Verification items for the finished model (mm, model axes). Face numbers are marked on the shaded views. A direction names the side the tool comes from. Coordinates: 2 decimals unless noted, no trailing zeros. Order: outer loops, then holes, each group sorted by start corner. A loop starts at its lowest first (then second) coordinate and runs counter-clockwise, first axis right, second up. Notation, with made-up numbers: M 7,-11 L 48,-11 A19 cw 48,5 Z; hole C -28,2 d4. An arc over 180 degrees is marked long. Use one line per item in the form item = value. Start each with the question number.
```python
from build123d import *

# Parameters (mm, degrees)
F1_DEPTH = 12
F0_W     = 22.75
F0_H     = 12
F2_DEPTH = 29
F3_DEPTH = 8
F4_W     = 10
F4_H     = 4.5
F5_DEPTH = 5.5


with BuildPart() as f1:
    # F0 (on Top) → F1 (new body)
    with BuildSketch(Plane.XY):
        with BuildLine():
            Line((37.5, -50), (34.2948445635, -50))
            ThreePointArc((34.2948445635, -50), (37.0207144417, -53.2303243355), (39.4433779545, -56.6938577061))
            ThreePointArc((39.4433779545, -56.6938577061), (37.9956721228, -53.4851272883), (37.5, -50))
        make_face()
        with BuildLine():
            Line((-34.2948445635, -50), (-37.5, -50))
            ThreePointArc((-37.5, -50), (-37.9956721876, -53.4851275115), (-39.4433782034, -56.6938580986))
            ThreePointArc((-39.4433782034, -56.6938580986), (-37.0207145834, -53.2303245197), (-34.2948445635, -50))
        make_face()
        with BuildLine():
            ThreePointArc((-39.443378119, 56.6938579655), (-37.9956721656, 53.4851274358), (-37.5, 50))
            Line((-37.5, 50), (-34.2948445635, 50))
            ThreePointArc((-34.2948445635, 50), (-37.0207145354, 53.2303244572), (-39.443378119, 56.6938579655))
        make_face()
        with BuildLine():
            Line((50, -34.2948445635), (50, -37.5))
            ThreePointArc((50, -37.5), (53.4851274351, -37.9956721654), (56.6938579643, -39.4433781183))
            ThreePointArc((56.6938579643, -39.4433781183), (53.2303244566, -37.020714535), (50, -34.2948445635))
        make_face()
        with BuildLine():
            Line((50, 37.5), (50, 34.2948445635))
            ThreePointArc((50, 34.2948445635), (53.2303242081, 37.0207143438), (56.6938574347, 39.4433777825))
            ThreePointArc((56.6938574347, 39.4433777825), (53.485127134, 37.995672078), (50, 37.5))
        make_face()
        with BuildLine():
            ThreePointArc((-56.6938576889, -39.4433779436), (-53.4851272786, -37.9956721199), (-50, -37.5))
            Line((-50, -37.5), (-50, -34.2948445635))
            ThreePointArc((-50, -34.2948445635), (-53.2303243274, -37.0207144356), (-56.6938576889, -39.4433779436))
        make_face()
        with BuildLine():
            ThreePointArc((-56.6938579169, 39.4433780882), (-53.2303244344, 37.0207145179), (-50, 34.2948445635))
            Line((-50, 34.2948445635), (-50, 37.5))
            ThreePointArc((-50, 37.5), (-53.4851274082, 37.9956721576), (-56.6938579169, 39.4433780882))
        make_face()
        with BuildLine():
            ThreePointArc((37.5, 50), (41.1611652352, 41.1611652352), (50, 37.5))
            Line((50, 37.5), (50, 44))
            ThreePointArc((50, 44), (45.7573593129, 45.7573593129), (44, 50))
            Line((44, 50), (37.5, 50))
        make_face()
        with BuildLine():
            Line((50, 44), (50, 37.5))
            ThreePointArc((50, 37.5), (53.485127134, 37.995672078), (56.6938574347, 39.4433777825))
            ThreePointArc((56.6938574347, 39.4433777825), (60.952698707, 43.9760153525), (62.5, 50))
            ThreePointArc((62.5, 50), (53.4152371074, 62.0243983426), (39.3662151199, 56.5705874261))
            ThreePointArc((39.3662151199, 56.5705874261), (37.9756016574, 53.4152371074), (37.5, 50))
            Line((37.5, 50), (44, 50))
            ThreePointArc((44, 50), (50, 56), (56, 50))
            ThreePointArc((56, 50), (54.2426406871, 45.7573593129), (50, 44))
        make_face()
        with BuildLine():
            Line((44, -50), (37.5, -50))
            ThreePointArc((37.5, -50), (37.9956721228, -53.4851272883), (39.4433779545, -56.6938577061))
            ThreePointArc((39.4433779545, -56.6938577061), (53.4851272883, -62.0043278772), (62.5, -50))
            ThreePointArc((62.5, -50), (60.9526988581, -43.9760156272), (56.6938579643, -39.4433781183))
            ThreePointArc((56.6938579643, -39.4433781183), (53.4851274351, -37.9956721654), (50, -37.5))
            Line((50, -37.5), (50, -44))
            ThreePointArc((50, -44), (54.2426406871, -45.7573593129), (56, -50))
            ThreePointArc((56, -50), (50, -56), (44, -50))
        make_face()
        with BuildLine():
            ThreePointArc((-39.4433782034, -56.6938580986), (-37.9956721876, -53.4851275115), (-37.5, -50))
            Line((-37.5, -50), (-44, -50))
            ThreePointArc((-44, -50), (-54.2426406871, -54.2426406871), (-50, -44))
            Line((-50, -44), (-50, -37.5))
            ThreePointArc((-50, -37.5), (-53.4851272786, -37.9956721199), (-56.6938576889, -39.4433779436))
            ThreePointArc((-56.6938576889, -39.4433779436), (-58.8388349363, -58.8388345933), (-39.4433782034, -56.6938580986))
        make_face()
        with BuildLine():
            ThreePointArc((-56.6938579169, 39.4433780882), (-53.4851274082, 37.9956721576), (-50, 37.5))
            Line((-50, 37.5), (-50, 44))
            ThreePointArc((-50, 44), (-54.2426406871, 54.2426406871), (-44, 50))
            Line((-44, 50), (-37.5, 50))
            ThreePointArc((-37.5, 50), (-37.9956721656, 53.4851274358), (-39.443378119, 56.6938579655))
            ThreePointArc((-39.443378119, 56.6938579655), (-58.8388347851, 58.8388347445), (-56.6938579169, 39.4433780882))
        make_face()
        with BuildLine():
            Line((22.75, 12), (22.75, 0))
            Line((22.75, 0), (35, 0))
            ThreePointArc((35, 0), (38.9140035649, 18.7158780427), (50, 34.2948445635))
            Line((50, 34.2948445635), (50, 37.5))
            ThreePointArc((50, 37.5), (41.1611652352, 41.1611652352), (37.5, 50))
            Line((37.5, 50), (34.2948445635, 50))
            ThreePointArc((34.2948445635, 50), (18.7158780427, 38.9140035649), (0, 35))
            Line((0, 35), (0, 12))
            Line((0, 12), (22.75, 12))
        make_face()
        with BuildLine():
            ThreePointArc((0, -35), (18.7158780427, -38.9140035649), (34.2948445635, -50))
            Line((34.2948445635, -50), (37.5, -50))
            ThreePointArc((37.5, -50), (41.1611652352, -41.1611652352), (50, -37.5))
            Line((50, -37.5), (50, -34.2948445635))
            ThreePointArc((50, -34.2948445635), (38.9140035649, -18.7158780427), (35, 0))
            Line((35, 0), (22.75, 0))
            Line((22.75, 0), (22.75, -12))
            Line((22.75, -12), (0, -12))
            Line((0, -12), (0, -35))
        make_face()
        with BuildLine():
            ThreePointArc((-50, -37.5), (-41.1611652352, -41.1611652352), (-37.5, -50))
            Line((-37.5, -50), (-34.2948445635, -50))
            ThreePointArc((-34.2948445635, -50), (-18.7158780427, -38.9140035649), (0, -35))
            Line((0, -35), (0, -12))
            Line((0, -12), (-22.75, -12))
            Line((-22.75, -12), (-22.75, 0))
            Line((-22.75, 0), (-35, 0))
            ThreePointArc((-35, 0), (-38.9140035649, -18.7158780427), (-50, -34.2948445635))
            Line((-50, -34.2948445635), (-50, -37.5))
        make_face()
        with BuildLine():
            Line((-50, 37.5), (-50, 34.2948445635))
            ThreePointArc((-50, 34.2948445635), (-38.9140035649, 18.7158780427), (-35, 0))
            Line((-35, 0), (-22.75, 0))
            Line((-22.75, 0), (-22.75, 12))
            Line((-22.75, 12), (0, 12))
            Line((0, 12), (0, 35))
            ThreePointArc((0, 35), (-18.7158780427, 38.9140035649), (-34.2948445635, 50))
            Line((-34.2948445635, 50), (-37.5, 50))
            ThreePointArc((-37.5, 50), (-41.1611652352, 41.1611652352), (-50, 37.5))
        make_face()
        with BuildLine():
            Line((-44, -50), (-37.5, -50))
            ThreePointArc((-37.5, -50), (-41.1611652352, -41.1611652352), (-50, -37.5))
            Line((-50, -37.5), (-50, -44))
            ThreePointArc((-50, -44), (-45.7573593129, -45.7573593129), (-44, -50))
        make_face()
        with BuildLine():
            Line((-50, 44), (-50, 37.5))
            ThreePointArc((-50, 37.5), (-41.1611652352, 41.1611652352), (-37.5, 50))
            Line((-37.5, 50), (-44, 50))
            ThreePointArc((-44, 50), (-45.7573593129, 45.7573593129), (-50, 44))
        make_face()
        with BuildLine():
            ThreePointArc((50, -37.5), (41.1611652352, -41.1611652352), (37.5, -50))
            Line((37.5, -50), (44, -50))
            ThreePointArc((44, -50), (45.7573593129, -45.7573593129), (50, -44))
            Line((50, -44), (50, -37.5))
        make_face()
        with BuildLine():
            ThreePointArc((39.2932775844, 56.4586962355), (36.935506218, 53.1198826695), (34.2948445635, 50))
            Line((34.2948445635, 50), (37.5, 50))
            ThreePointArc((37.5, 50), (37.9756016574, 53.4152371074), (39.3662151199, 56.5705874261))
            Line((39.3662151199, 56.5705874261), (39.2932775844, 56.4586962355))
        make_face()
    extrude(amount=F1_DEPTH)

    # F0 (on Top) → F2 (join)
    with BuildSketch(Plane.XY):
        with Locations((-11.375, 6)):
            Rectangle(F0_W, F0_H)
        with Locations((11.375, 6)):
            Rectangle(F0_W, F0_H)
        with Locations((11.375, -6)):
            Rectangle(F0_W, F0_H)
        with Locations((-11.375, -6)):
            Rectangle(F0_W, F0_H)
    extrude(amount=F2_DEPTH)

    # F0 (on Top) → F3 (join)
    with BuildSketch(Plane.XY):
        with BuildLine():
            ThreePointArc((-44, 50), (-54.2426406871, 54.2426406871), (-50, 44))
            Line((-50, 44), (-50, 47.5))
            ThreePointArc((-50, 47.5), (-51.767766953, 51.767766953), (-47.5, 50))
            Line((-47.5, 50), (-44, 50))
        make_face()
        with BuildLine():
            Line((-50, 47.5), (-50, 44))
            ThreePointArc((-50, 44), (-45.7573593129, 45.7573593129), (-44, 50))
            Line((-44, 50), (-47.5, 50))
            ThreePointArc((-47.5, 50), (-48.232233047, 48.232233047), (-50, 47.5))
        make_face()
        with BuildLine():
            Line((50, 47.5), (50, 44))
            ThreePointArc((50, 44), (54.2426406871, 45.7573593129), (56, 50))
            ThreePointArc((56, 50), (50, 56), (44, 50))
            Line((44, 50), (47.5, 50))
            ThreePointArc((47.5, 50), (50, 52.5), (52.5, 50))
            ThreePointArc((52.5, 50), (51.767766953, 48.232233047), (50, 47.5))
        make_face()
        with BuildLine():
            ThreePointArc((44, 50), (45.7573593129, 45.7573593129), (50, 44))
            Line((50, 44), (50, 47.5))
            ThreePointArc((50, 47.5), (48.232233047, 48.232233047), (47.5, 50))
            Line((47.5, 50), (44, 50))
        make_face()
        with BuildLine():
            ThreePointArc((50, -44), (45.7573593129, -45.7573593129), (44, -50))
            Line((44, -50), (47.5, -50))
            ThreePointArc((47.5, -50), (48.232233047, -48.232233047), (50, -47.5))
            Line((50, -47.5), (50, -44))
        make_face()
        with BuildLine():
            Line((47.5, -50), (44, -50))
            ThreePointArc((44, -50), (50, -56), (56, -50))
            ThreePointArc((56, -50), (54.2426406871, -45.7573593129), (50, -44))
            Line((50, -44), (50, -47.5))
            ThreePointArc((50, -47.5), (51.767766953, -48.232233047), (52.5, -50))
            ThreePointArc((52.5, -50), (50, -52.5), (47.5, -50))
        make_face()
        with BuildLine():
            Line((-47.5, -50), (-44, -50))
            ThreePointArc((-44, -50), (-45.7573593129, -45.7573593129), (-50, -44))
            Line((-50, -44), (-50, -47.5))
            ThreePointArc((-50, -47.5), (-48.232233047, -48.232233047), (-47.5, -50))
        make_face()
        with BuildLine():
            ThreePointArc((-50, -44), (-54.2426406871, -54.2426406871), (-44, -50))
            Line((-44, -50), (-47.5, -50))
            ThreePointArc((-47.5, -50), (-51.767766953, -51.767766953), (-50, -47.5))
            Line((-50, -47.5), (-50, -44))
        make_face()
    extrude(amount=F3_DEPTH)

    # F4 (on face) → F5 (cut)
    with BuildSketch(Plane.XZ.offset(12)):
        with Locations((-14, 19.25)):
            Rectangle(F4_W, F4_H)
        with Locations((14, 19.25)):
            Rectangle(F4_W, F4_H)
    extrude(amount=-F5_DEPTH, mode=Mode.SUBTRACT)


solid = f1.part
```
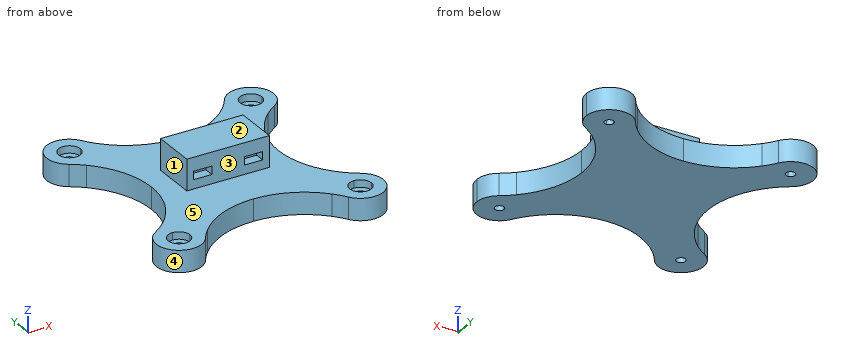
1. Material ranges on line 1 along X through (y, z) = (50, 9.05); line 2 along X through (y, z) = (-50, 4), recorded low to high.
2. Cross-section at A-A on z = 18.75. Enter the section's corners in (x, y).
3. Depth check by flat-ended pin: P1, Ø15.5, axis at x = -50, y = 50, coming from the +Z side; P2, Ø8.5, axis at x = 0, z = 17, coming from the -Y side; P3, Ø5, axis at y = 2, z = 16.5, coming from the -X side; P4, Ø4.5, axis at x = -50, y = -50, coming from the +Z side. Enter the tip coordinate at first touch or a pass-through.
4. Cross-section at B-B on y = 41.5. Enter the section's corners in (x, z), and give its area (3 significant figures).
5. Tool access check on the marked faces 1 and 2. Record the directions out of +Z, -Z, +X, -X, +Y, -Y that give a thin tool (end or side, any length) a straight path to the whole face; none if there is none.
6. Cross-section at D-D on x = 6.5. Enter the section's corners in (y, z), and give its area (3 significant figures).
7. Cross-section at C-C on y = 2.5. Enter the section's corners in (x, z), and give its area (3 significant figures).
8. Release check for a two-part mould opening along Y. For the marked faces 3, 4 and 5 record: pulls with the +Y half, pulls with the -Y half, needs draft (parallel to the pull), parting line crosses it, or undercut.
Final values:
q1.line_1 = -62.5 to -56, -44 to -34.29, 34.29 to 44, 56 to 62.5
q1.line_2 = -62.5 to -52.5, -47.5 to -34.29, 34.29 to 47.5, 52.5 to 62.5
q2.outline = M -22.75,-12 L -19,-12 L -19,-6.5 L -9,-6.5 L -9,-12 L 9,-12 L 9,-6.5 L 19,-6.5 L 19,-12 L 22.75,-12 L 22.75,12 L -22.75,12 Z
q3.P1 = 12
q3.P2 = -12
q3.P3 = -22.75
q3.P4 = through
q4.outline = M -59.17,0 L -23.77,0 L -23.77,12 L -59.17,12 Z; M 23.77,0 L 59.17,0 L 59.17,12 L 23.77,12 Z
q4.area = 850 mm2
q5.face_1 = +Z, -X, +Y, -Y
q5.face_2 = +Z, +X, -X, +Y, -Y
q6.outline = M -35.45,0 L 35.45,0 L 35.45,12 L 12,12 L 12,29 L -12,29 L -12,12 L -35.45,12 Z
q6.area = 1,260 mm2
q7.outline = M -35.07,0 L 35.07,0 L 35.07,12 L 22.75,12 L 22.75,29 L -22.75,29 L -22.75,12 L -35.07,12 Z
q7.area = 1,620 mm2
q8.face_3 = pulls with the -Y half
q8.face_4 = undercut
q8.face_5 = needs draft
